Drawing for the job (mm, zero at the part's lowest x, y, z). A direction names the side the tool comes from. Give positions to 0.01 mm unless a question says otherwise; leave off trailing zeros. Order: outer loops, then holes, each group sorted by start corner. A loop starts at its lowest first (then second) coordinate and runs counter-clockwise, first axis right, second up. Notation, with made-up numbers: M 35.5,26 L 77.5,26 A21 cw 77.5,37 Z; hole C 75,58 d1. An arc over 180 degrees is marked long. Answer as a JSON object with one key per item and string values.
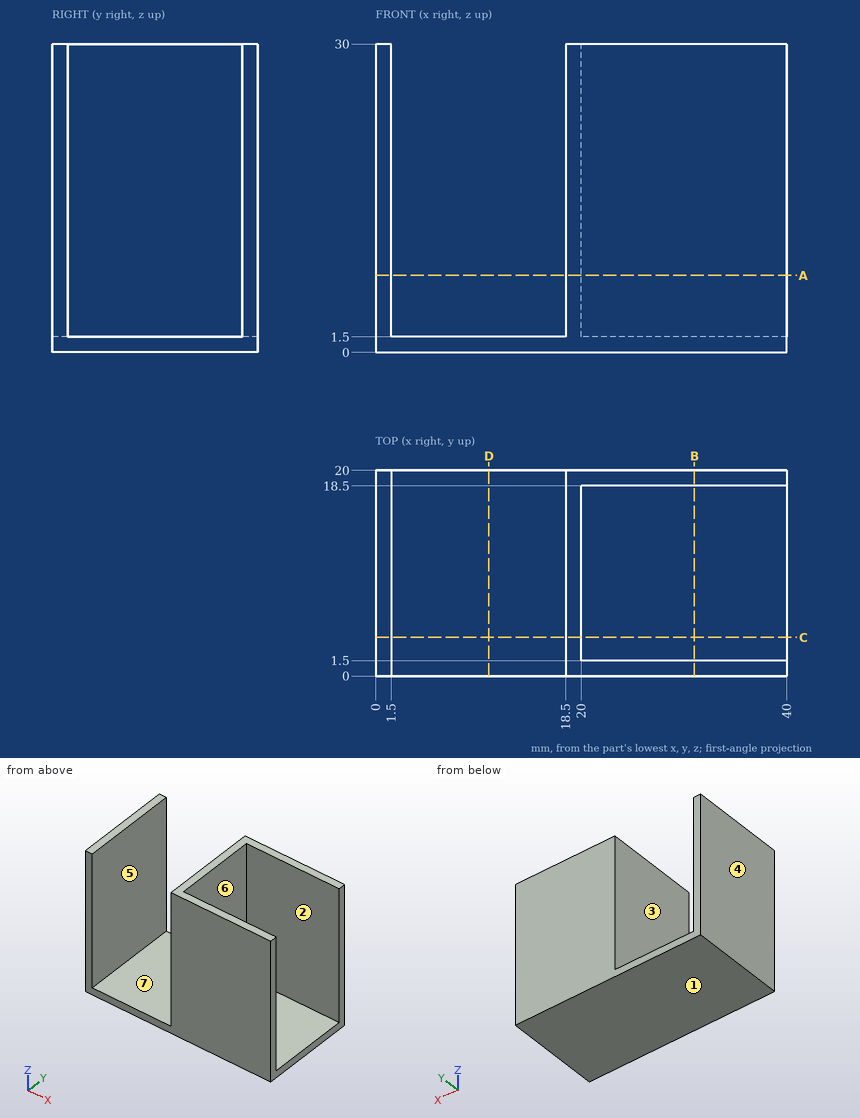
1. Two-plate mould, pull along X, no slides. Class the marked faces 4, 5, 6 and 7: +X half, -X half, draft (parallel to the pull), parting line (faces both ways), or undercut.
Worked answers:
{"face 4": "-X half", "face 5": "undercut", "face 6": "+X half", "face 7": "undercut"}
2. Cut at B-B on x = 31. Give the cut face in (y, z).
Worked answers:
{"outline": "M 0,0 L 20,0 L 20,30 L 18.5,30 L 18.5,1.5 L 1.5,1.5 L 1.5,30 L 0,30 Z"}
3. Cut at D-D on x = 11. Give the cut face in (y, z).
Worked answers:
{"outline": "M 0,0 L 20,0 L 20,1.5 L 0,1.5 Z"}
4. Cut at A-A on z = 7.5. Give the cut face in (x, y).
Worked answers:
{"outline": "M 0,0 L 1.5,0 L 1.5,20 L 0,20 Z; M 18.5,0 L 40,0 L 40,1.5 L 20,1.5 L 20,18.5 L 40,18.5 L 40,20 L 18.5,20 Z"}
5. Pin check, flat tips, straight feed: P1, Ø12, axis at y = 5, z = 15, coming from the -X side; P2, Ø2, axis at y = 10.5, z = 12, coming from the +X side; P3, Ø5, axis at x = 12, y = 11, coming from the +Z side. Stop position of each tip, or through.
Worked answers:
{"P1": "stops at x = 0", "P2": "stops at x = 20", "P3": "stops at z = 1.5"}
6. Probe line 1 along Y through (x, z) = (23, 10.75); line 2 along X through (y, z) = (19.25, 27.5). List the from-to ranges inside material, lowest first.
Worked answers:
{"line 1": "y = 0 to 1.5, 18.5 to 20", "line 2": "x = 0 to 1.5, 18.5 to 40"}
7. Cut at C-C on y = 3.75. Give the cut face in (x, z).
Worked answers:
{"outline": "M 0,0 L 40,0 L 40,1.5 L 20,1.5 L 20,30 L 18.5,30 L 18.5,1.5 L 1.5,1.5 L 1.5,30 L 0,30 Z"}
8. Which spindle directions (+Z, -Z, +X, -X, +Y, -Y) get a long thin tool onto all of the face, cutting with end or side? Do the marked faces 1, 2 and 3. Say none if no direction does.
Worked answers:
{"face 1": "-Z, +X, -X, +Y, -Y", "face 2": "+Z, +X", "face 3": "+Z, +Y, -Y"}
